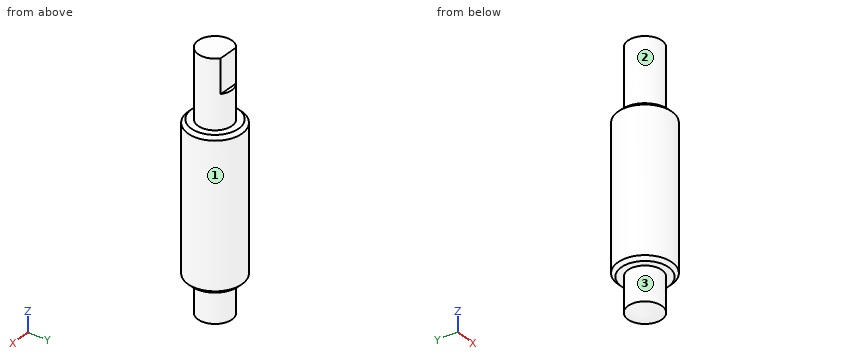
```python
from build123d import *

# Parameters (mm, degrees)
CUT_EXTRUDE1_START = -10
CUT_EXTRUDE1_DEPTH = 10


with BuildPart() as part:
    # Sketch1 → Revolve1 (revolve)
    with BuildSketch(Plane(origin=(0, 0, 0), x_dir=(1, 0, 0), z_dir=(0, 1, 0)), mode=Mode.PRIVATE) as revolve1_sk:
        Polygon((0, 74), (0, 0), (5, 0), (5, 20), (7, 20), (8, 21), (8, 63), (7, 64), (5, 64), (5, 74), (0, 76.886751346), align=None)
    revolve(revolve1_sk.sketch.rotate(Axis((0, 0, -74), (0, 0, 1)), 180), axis=Axis((0, 0, -74), (0, 0, 1)))

    # Sketch2 → Cut-Extrude1 (cut)
    with BuildSketch(Plane.XY.offset(CUT_EXTRUDE1_START)):
        with BuildLine():
            Line((-3, 4), (3, 4))
            ThreePointArc((3, 4), (0, 5), (-3, 4))
        make_face()
    extrude(amount=CUT_EXTRUDE1_DEPTH, mode=Mode.SUBTRACT)


solid = part.part
```
The model under review builds one solid part; all positions refer to its coordinate system, in mm. Face numbers are marked on the shaded views. A direction names the side the tool comes from. Round coordinates to 2 decimals unless told otherwise and drop trailing zeros. Order: outer loops, then holes, each group sorted by start corner. A loop starts at its lowest first (then second) coordinate and runs counter-clockwise, first axis right, second up. Notation, with made-up numbers: (79.25, -37.5) -> (121.25, -37.5) arc R17 ccw to (121.25, -4.5) -> close; hole circle Ø11 at (-17, 40). An arc over 180 degrees is marked (long way). One line per item, written item: value. Start each with the question number.
Q1. Clearance check with flat-ended pins moving along their axes: pin 1 Ø0.5 at (x, y) = (1.5, 4.5) entering from +Z; pin 2 Ø6 at (y, z) = (-4.5, -61) entering from +X; pin 3 Ø1 at (x, y) = (-4, 2) entering from -Z. State where each tip first meets the part, or that it passes through.
Q2. Take a section at A-A (z = -57). Write out the cut boundary in (x, y).
Q3. Wall thickness on line 1 (Y direction, x = -0.5, z = -57); line 2 (Z direction, x = 6.75, y = 0.5); line 3 (X direction, y = 4, z = -12.5): over which ranges is each line inside the solid? List them lowest first.
Q4. Take a section at B-B (z = -18.5). Write out the cut boundary in (x, y), and give its area (3 significant figures).
Q5. Machinability: for the marked faces 1, 2 and 3, which of the approach directions +Z, -Z, +X, -X, +Y, -Y give a long, thin tool a straight path to every point of the face, cutting with its end or side? Answer none if there is none.
Reported:
1. pin 1: stops at z = -10
1. pin 2: stops at x = 7.86
1. pin 3: stops at z = -74.59
2. outline: circle Ø16 at (0, 0)
3. line 1: y = -7.98 to 7.98
3. line 2: z = -64 to -20
3. line 3: x = -3 to 3
4. outline: circle Ø10 at (0, 0)
4. area: 78.5 mm2
5. face 1: +Z, -Z
5. face 2: +Z
5. face 3: -Z
